Verification items for the finished model (mm, model axes). Face numbers are marked on the shaded views. Round coordinates to 2 decimals unless told otherwise and drop trailing zeros. Order: outer loops, then holes, each group sorted by start corner. A loop starts at its lowest first (then second) coordinate and runs counter-clockwise, first axis right, second up. Notation, with made-up numbers: M 17,33.5 L 75,33.5 A12 ccw 75,54.5 Z; hole C 73.25,88 d9. An arc over 180 degrees is marked long. Use CSV: the item, a comma, the result in double quotes. Start each with the question number.
Q1. Sectioned sample at A-A (x = 37.5). Enter the section's corners in (y, z), and give its area (3 significant figures).
Q2. Scan lines: line 1 (X direction, y = 1.25, z = -55); line 2 (Z direction, x = 68.5, y = 4.15); line 3 (Z direction, x = 10, y = 1). Record each from-to range of solid material in increasing order.
Q3. Gauge pin test, flat end, axial feed: pin 1 Ø18.5 at (x, z) = (68.791, -21.209) entering from -Y. Record the tip position at first contact, or that the pin passes through.
Q4. Sectioned sample at C-C (y = 1.2). State how many separate pieces and enclosed holes the cut face has, and give its area (3 significant figures).
Q5. Sectioned sample at B-B (z = -55). Enter the section's corners in (x, y), and give its area (3 significant figures).
Q6. Sectioned sample at D-D (x = 61.5). Enter the section's corners in (y, z), and give its area (3 significant figures).
Q7. Mould release check, pull along Z, two halves, no side actions. Record for the marked faces 1 and 2: +Z half, -Z half, draft (parallel to the pull), parting line (faces both ways), or undercut.
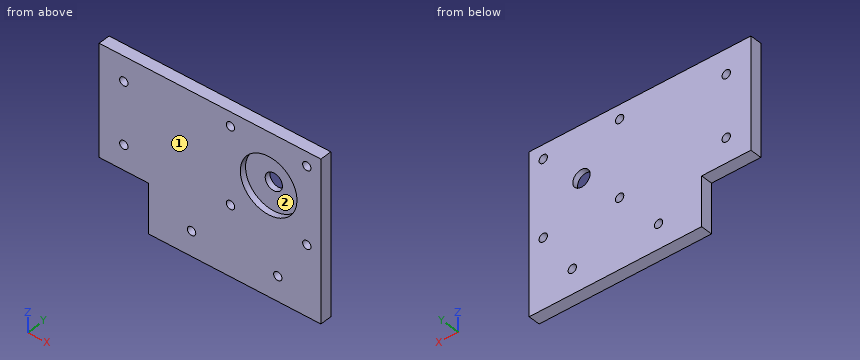
```python
from build123d import *

# Parameters (mm, degrees)
BOSS_EXTRUDE1_DEPTH      = 4.7625
F_7_0_7_DIAMETER_HOLE1_D = 7
SKETCH12_R               = 11.5
CUT_EXTRUDE1_DEPTH       = 2.5
M3_CLEARANCE_HOLE1_D     = 3.4


with BuildPart() as part:
    # Sketch1 → Boss-Extrude1 (new body)
    with BuildSketch(Plane(origin=(0, 0, 0), x_dir=(1, 0, 0), z_dir=(0, 1, 0))):
        Polygon((0, 0), (0, 45), (20, 45), (20, 65), (90, 65), (90, 0), align=None)
    extrude(amount=BOSS_EXTRUDE1_DEPTH)

    # Ø7.0 (7) Diameter Hole1 (through all)
    with Locations(Plane(origin=(0, 0, 0), x_dir=(-1, 0, 0), z_dir=(0, -1, 0))):
        with Locations((-68.791, 21.209)):
            Hole(F_7_0_7_DIAMETER_HOLE1_D / 2)

    # Sketch12 → Cut-Extrude1 (cut)
    with BuildSketch(Plane.XZ):
        with Locations(Location((68.791, -21.209, 0), (0, 0, 270))):
            Circle(SKETCH12_R)
    extrude(amount=-CUT_EXTRUDE1_DEPTH, mode=Mode.SUBTRACT)

    # M3 Clearance Hole1 (through all)
    with Locations(Plane(origin=(0, 0, 0), x_dir=(-1, 0, 0), z_dir=(0, -1, 0))):
        with Locations((-10, 10), (-10, 35), (-37.5, 55), (-72.5, 55), (-84.291, 36.709), (-84.291, 5.709), (-53.291, 5.709), (-53.291, 36.709)):
            Hole(M3_CLEARANCE_HOLE1_D / 2)


solid = part.part
```
Verdict:
1,outline,"M 0,-65 L 4.76,-65 L 4.76,-56.7 L 0,-56.7 Z; M 0,-53.3 L 4.76,-53.3 L 4.76,0 L 0,0 Z"
1,area,"293 mm²"
2,line 1,"x = 20 to 35.8, 39.2 to 70.8, 74.2 to 90"
2,line 2,"z = -65 to -24.7, -17.72 to 0"
2,line 3,"z = -45 to -36.7, -33.3 to -11.7, -8.3 to 0"
3,pin 1,"stops at y = 2.5"
4,separate pieces,"1"
4,enclosed holes,"9"
4,area,"4,960 mm²"
5,outline,"M 20,0 L 35.8,0 L 35.8,4.76 L 20,4.76 Z; M 39.2,0 L 70.8,0 L 70.8,4.76 L 39.2,4.76 Z; M 74.2,0 L 90,0 L 90,4.76 L 74.2,4.76 Z"
5,area,"301 mm²"
6,outline,"M 0,-65 L 4.76,-65 L 4.76,0 L 0,0 L 0,-12.32 L 2.5,-12.32 L 2.5,-30.1 L 0,-30.1 Z"
6,area,"265 mm²"
7,face 1,"draft"
7,face 2,"undercut"
